Autodesk Inventor part; units mm, degrees
ref_plane "YZ Plane" through (0, 0, 0) normal (1, 0, 0) x (0, 1, 0)
ref_plane "XZ Plane" through (0, 0, 0) normal (0, 1, 0) x (-1, 0, 0)
ref_plane "XY Plane" through (0, 0, 0) normal (0, 0, 1) x (1, 0, 0)
sketch "Sketch1" plane through (0, 0, 0) normal (0, 1, 0) x (-1, 0, 0)
  line L0 (-2.5, 18) -> (2.5, 18)
  line L1 (4.5, 16) -> (4.5, -16)
  line L2 (2.5, -18) -> (-2.5, -18)
  line L3 (-4.5, -16) -> (-4.5, 16)
  line L4 (-4.5, 18) -> (4.5, -18) construction
  line L5 (4.5, 18) -> (-4.5, -18) construction
  circle A0 centre (0, 14) radius 1.9
  line L6 (0, 14) -> (0, -14) construction
  circle A1 centre (0, -14) radius 1.9
  arc A2 (4.5, 16) -> (2.5, 18) centre (2.5, 16) ccw
  arc A3 (2.5, -18) -> (4.5, -16) centre (2.5, -16) ccw
  arc A4 (-4.5, -16) -> (-2.5, -18) centre (-2.5, -16) ccw
  arc A5 (-2.5, 18) -> (-4.5, 16) centre (-2.5, 16) ccw
  point P0 (0, 0)
  point P1 (0, 0)
  dimension "d0" = 3.8
  dimension "d1" = 28
  dimension "d2" = 36
  dimension "d3" = 9
  dimension "d4" = 2
  dimension "d5" = 2
  dimension "d6" = 2
extrude "Extrusion1" add sketch "Sketch1" along normal blind 6
sketch "Sketch2" plane through (4.5, 0, 16) normal (1, 0, 0) x (0, 0, -1)
  line L0 (32, 6) -> (0, 6) construction
  line L1 (5.5, 6) -> (10.267, 2)
  line L2 (10.267, 2) -> (16, 2)
  line L3 (16, 0) -> (16, 6) construction
  line L4 (16, 2) -> (16, 6)
  line L5 (5.5, 6) -> (16, 6)
  line L6 (0, 0) -> (32, 0)
  line L7 (26.5, 6) -> (21.733, 2)
  line L8 (21.733, 2) -> (16, 2)
  line L9 (26.5, 6) -> (16, 6)
  dimension "d9" = 2
  dimension "d10" = 10.5
  dimension "d11" = 40
extrude "Extrusion2" cut sketch "Sketch2" against normal through all
sketch "Sketch3" plane through (0, 0, 0) normal (0, -1, 0) x (1, 0, 0)
  line L0 (4.5, 16) -> (4.5, -16) construction
  line L1 (4.5, 15) -> (3.5, 13.2679)
  line L2 (3.5, 13.2679) -> (3.5, 6.7321)
  line L3 (3.5, 6.7321) -> (4.5, 5)
  line L4 (4.5, 15) -> (4.5, 5)
  line L5 (-2.5, 18) -> (2.5, 18)
  point P0 (0, 0)
  dimension "d14" = 150
  dimension "d15" = 150
  dimension "d16" = 1
  dimension "d17" = 3
  dimension "d18" = 10
extrude "Extrusion3" cut sketch "Sketch3" against normal through all
properties part number "CH_01_0033_syringe_pump_nut_mount" material "ABS Plastic"
Read the model definition and answer for the solid it produces. Units are mm, in the model's axes. A direction names the side the tool comes from. Give positions to 0.01 mm unless a question says otherwise; leave off trailing zeros. Write each loop counter-clockwise with the first axis right and the second up, starting at its lowest first coordinate (ties: lowest second). Pieces come first, ordered by that corner, then holes. Notation, with made-up numbers: (16.25, -35.75) - (47.25, -35.75) arc R29 cw to (47.25, 1.25) - close; hole circle Ø2 at (33, -7.75). An arc over 180 degrees is marked (long way). Answer in a Markdown table with one row per item. Add a question column.
Item 1: Section C-C, the plane z = -14 is taken. Write down the section's boundary in (x, y).
Item 2: Flat-ended cylindrical pins translate along their axes: P1, Ø1, axis at x = 1, z = -1, coming from the +Y side; P2, Ø1.5, axis at x = 3, z = -6, coming from the +Y side; P3, Ø3.5, axis at x = 0, z = 14, coming from the -Y side. Find the tip coordinate at first contact, or state that the pin passes through.
Item 3: Section D-D, the plane x = 0 is taken. Write down the section's boundary in (y, z), and give its area (3 significant figures).
Item 4: Determine the mould class of faces 4 (the face through (0, 0, 0)), 5 (the face through (3.99, 1.08, 5.88)), 6 (the face through (-3.9, 2.96, 17.43)) for opening direction Z: pulls with the +Z half, pulls with the -Z half, needs draft (parallel to the pull), parting line crosses it, or undercut.
Item 5: Section A-A, the plane y = 1 is taken. Write down the section's boundary in (x, z).
Item 6: Section B-B, the plane y = 3.5 is taken. Write down the section's boundary in (x, z).
Item 7: A tool of negligible diameter and unlimited length cuts with its end or side. For faces 1 (the face through (4.01, 2.96, 14.15)), 2 (the face through (4.5, 2, -8)), 3 (the face through (-0.15, 4.03, 8.15)), from which of +Z, -Z, +X, -X, +Y, -Y can it reach the whole face along a straight path? Write none if from no direction.
Item 8: Find the intervals of material crossed by L1, parallel to Z at x = 0, y = 1.5; L2, parallel to Z at x = 0, y = 2.2; L3, parallel to Z at x = 0, y = 4.5, in increasing order.
Recorded:
| question | item | result |
|---|---|---|
| 1 | outline | (-4.5, 0) - (-1.9, 0) - (-1.9, 6) - (-4.5, 6) - close; (1.9, 0) - (4.5, 0) - (4.5, 6) - (1.9, 6) - close |
| 2 | P1 | stops at y = 2 |
| 2 | P2 | stops at y = 2.85 |
| 2 | P3 | passes through |
| 3 | outline | (0, -18) - (6, -18) - (6, -15.9) - (0, -15.9) - close; (0, -12.1) - (6, -12.1) - (6, -10.5) - (2, -5.73) - (2, 5.73) - (6, 10.5) - (6, 12.1) - (0, 12.1) - close; (0, 15.9) - (6, 15.9) - (6, 18) - (0, 18) - close |
| 3 | area | 105 mm2 |
| 4 | face 4 | needs draft |
| 4 | face 5 | undercut |
| 4 | face 6 | pulls with the +Z half |
| 5 | outline | (-4.5, -16) arc R2 ccw to (-2.5, -18) - (2.5, -18) arc R2 ccw to (4.5, -16) - (4.5, 5) - (3.5, 6.73) - (3.5, 13.27) - (4.5, 15) - (4.5, 16) arc R2 ccw to (2.5, 18) - (-2.5, 18) arc R2 ccw to (-4.5, 16) - close; hole circle Ø3.8 at (0, -14); hole circle Ø3.8 at (0, 14) |
| 6 | outline | (-4.5, -16) arc R2 ccw to (-2.5, -18) - (2.5, -18) arc R2 ccw to (4.5, -16) - (4.5, -7.52) - (-4.5, -7.52) - close; (-4.5, 7.52) - (3.5, 7.52) - (3.5, 13.27) - (4.5, 15) - (4.5, 16) arc R2 ccw to (2.5, 18) - (-2.5, 18) arc R2 ccw to (-4.5, 16) - close; hole circle Ø3.8 at (0, -14); hole circle Ø3.8 at (0, 14) |
| 7 | face 1 | +X, +Y, -Y |
| 7 | face 2 | +Z, -Z, +X, +Y, -Y |
| 7 | face 3 | +X, -X, +Y |
| 8 | L1 | z = -18 to -15.9, -12.1 to 12.1, 15.9 to 18 |
| 8 | L2 | z = -18 to -15.9, -12.1 to -5.97, 5.97 to 12.1, 15.9 to 18 |
| 8 | L3 | z = -18 to -15.9, -12.1 to -8.71, 8.71 to 12.1, 15.9 to 18 |
